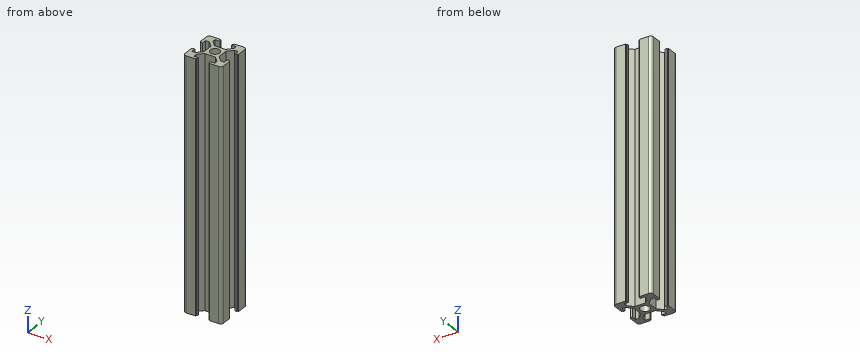
```python
from build123d import *

# Parameters (mm, degrees)
SKETCH_2_R      = 2.5
EXTRUDE_1_DEPTH = 130


with BuildPart() as part:
    # 草图2 → 凸台-拉伸1 (new body)
    with BuildSketch(Plane.XY):
        with BuildLine():
            Line((-3.6, 10), (-3.6, 9.5))
            Line((-3.6, 9.5), (-3.1, 9.5))
            Line((-3.1, 9.5), (-3.1, 8.5))
            Line((-3.1, 8.5), (-5.5, 8.5))
            Line((-5.5, 8.5), (-5.5, 6.65))
            Line((-5.5, 6.65), (-2.75, 3.9))
            Line((-2.75, 3.9), (2.75, 3.9))
            Line((2.75, 3.9), (5.5, 6.65))
            Line((5.5, 6.65), (5.5, 8.5))
            Line((5.5, 8.5), (3.1, 8.5))
            Line((3.1, 8.5), (3.1, 9.5))
            Line((3.1, 9.5), (3.6, 9.5))
            Line((3.6, 9.5), (3.6, 10))
            Line((3.6, 10), (8.5, 10))
            ThreePointArc((8.5, 10), (9.560660172, 9.560660172), (10, 8.5))
            Line((10, 8.5), (10, 3.6))
            Line((10, 3.6), (9.5, 3.6))
            Line((9.5, 3.6), (9.5, 3.1))
            Line((9.5, 3.1), (8.5, 3.1))
            Line((8.5, 3.1), (8.5, 5.5))
            Line((8.5, 5.5), (6.65, 5.5))
            Line((6.65, 5.5), (3.9, 2.75))
            Line((3.9, 2.75), (3.9, -2.75))
            Line((3.9, -2.75), (6.65, -5.5))
            Line((6.65, -5.5), (8.5, -5.5))
            Line((8.5, -5.5), (8.5, -3.1))
            Line((8.5, -3.1), (9.5, -3.1))
            Line((9.5, -3.1), (9.5, -3.6))
            Line((9.5, -3.6), (10, -3.6))
            Line((10, -3.6), (10, -8.5))
            ThreePointArc((10, -8.5), (9.560660172, -9.560660172), (8.5, -10))
            Line((8.5, -10), (3.6, -10))
            Line((3.6, -10), (3.6, -9.5))
            Line((3.6, -9.5), (3.1, -9.5))
            Line((3.1, -9.5), (3.1, -8.5))
            Line((3.1, -8.5), (5.5, -8.5))
            Line((5.5, -8.5), (5.5, -6.65))
            Line((5.5, -6.65), (2.75, -3.9))
            Line((2.75, -3.9), (-2.75, -3.9))
            Line((-2.75, -3.9), (-5.5, -6.65))
            Line((-5.5, -6.65), (-5.5, -8.5))
            Line((-5.5, -8.5), (-3.1, -8.5))
            Line((-3.1, -8.5), (-3.1, -9.5))
            Line((-3.1, -9.5), (-3.6, -9.5))
            Line((-3.6, -9.5), (-3.6, -10))
            Line((-3.6, -10), (-8.5, -10))
            ThreePointArc((-8.5, -10), (-9.560660172, -9.560660172), (-10, -8.5))
            Line((-10, -8.5), (-10, -3.6))
            Line((-10, -3.6), (-9.5, -3.6))
            Line((-9.5, -3.6), (-9.5, -3.1))
            Line((-9.5, -3.1), (-8.5, -3.1))
            Line((-8.5, -3.1), (-8.5, -5.5))
            Line((-8.5, -5.5), (-6.65, -5.5))
            Line((-6.65, -5.5), (-3.9, -2.75))
            Line((-3.9, -2.75), (-3.9, 2.75))
            Line((-3.9, 2.75), (-6.65, 5.5))
            Line((-6.65, 5.5), (-8.5, 5.5))
            Line((-8.5, 5.5), (-8.5, 3.1))
            Line((-8.5, 3.1), (-9.5, 3.1))
            Line((-9.5, 3.1), (-9.5, 3.6))
            Line((-9.5, 3.6), (-10, 3.6))
            Line((-10, 3.6), (-10, 8.5))
            ThreePointArc((-10, 8.5), (-9.560660172, 9.560660172), (-8.5, 10))
            Line((-8.5, 10), (-3.6, 10))
        make_face()
        Circle(SKETCH_2_R, mode=Mode.SUBTRACT)
    extrude(amount=EXTRUDE_1_DEPTH)


solid = part.part
```
Input: part model. Units: mm. Frame: model coordinates. Give positions to 0.01 mm unless a question says otherwise; leave off trailing zeros. Order: outer loops, then holes, each group sorted by start corner. A loop starts at its lowest first (then second) coordinate and runs counter-clockwise, first axis right, second up. Notation, with made-up numbers: (-17.75, 44.25) -> (27.25, 44.25) arc R20 ccw to (27.25, 65.25) -> close; hole circle Ø1 at (-15.75, 74.25). An arc over 180 degrees is marked (long way). Write each question's results on one line, items separated by ' | '. Start each with the question number.
Item 1: Line query: line 1 (X direction, y = 8, z = 109.5); line 2 (Y direction, x = 0, z = 33); line 3 (Y direction, x = -4, z = 74.5). Output: solid intervals per line, ascending.
Item 2: Contact query for flat-ended pins moving along their axis: P1, Ø0.6, axis at y = 9.5, z = 39, coming from the -X side; P2, Ø1.6, axis at x = 0, z = 63.5, coming from the +Y side; P3, Ø1.6, axis at y = 0, z = 92, coming from the +X side. Output: stop coordinate, or through.
Item 3: Cut plane A-A on x = 0. Return the cut outline in (y, z).
Established:
1) line 1: -10 to -5.5, 5.5 to 10 | line 2: -3.9 to -2.5, 2.5 to 3.9 | line 3: -10 to -8.5, -5.15 to -2.85, 2.85 to 5.15, 8.5 to 10
2) P1: x = -9.83 | P2: y = 3.9 | P3: x = 3.9
3) outline: (-3.9, 0) -> (-2.5, 0) -> (-2.5, 130) -> (-3.9, 130) -> close; (2.5, 0) -> (3.9, 0) -> (3.9, 130) -> (2.5, 130) -> close
